Could you check a few things on this model? Use its own coordinates, in mm. A direction names the side the tool comes from. Coordinates: 2 decimals unless noted, no trailing zeros. Order: outer loops, then holes, each group sorted by start corner. A loop starts at its lowest first (then second) coordinate and runs counter-clockwise, first axis right, second up. Notation, with made-up numbers: (75, 29) - (134, 29) arc R16 cw to (134, 44) - close; hole circle Ø3 at (75.25, 69). An arc over 180 degrees is marked (long way). Answer as a JSON object with one key per item and string values. Group by question number.
(1) We'd pull the mould along X, two halves only. Please class faces 1 (the flat face through (-0.775, 16, 1)), 2 (the flat face through (-16, -0.775, 1)), 3 (the cylindrical face through (25.275, 19.38, 0.986)): pulls with the +X half, pulls with the -X half, needs draft (parallel to the pull), parting line crosses it, or undercut.
(2) Imagine slicing it at A-A, the plane x = -7.5. Write out the boundary of the cut face in (y, z) (3 decimals), and give its area (3 significant figures).
(3) Imagine slicing it at B-B, the plane y = 25.5. Write out the boundary of the cut face in (x, z) (3 decimals).
(4) Please list where these lines run through material, in increasing order: probe 1 along Z at (x, y) = (22.5, 26); probe 2 along Z at (x, y) = (-0.5, -31.5); probe 3 along Y at (x, z) = (-28, 1.35) (3 decimals).
(5) Imagine slicing it at C-C, the plane z = 3.5. Write out the boundary of the cut face in (x, y), and give its area (3 significant figures).
(6) Which directions (+Z, -Z, +X, -X, +Y, -Y) give clear straight access to the entire face, cutting with the end or side of a thin tool? Please do faces 4 (the flat face through (-16, 0.775, 1)), 5 (the flat face through (10, 31, 2)), 6 (the flat face through (0.775, 0, 1)).
(7) Will these pins go through, and if not, where does the flat tip stop? P1, Ø1.2, axis at x = -11, z = 0.5, coming from the -Y side; P2, Ø2, axis at x = 27, z = 2, coming from the -Y side; P3, Ø1.2, axis at y = 18, z = 0.5, coming from the +X side.
from build123d import *

# Parameters (mm, degrees)
SKETCH1_R               = 34.5
BOSS_EXTRUDE1_DEPTH     = 4.5
SKETCH2_W               = 2.65
SKETCH2_H               = 2
CUT_EXTRUDE1_DEPTH      = 49.997448913
CUT_EXTRUDE1_DEPTH_BACK = 49.997448913
SKETCH4_W               = 1.55
SKETCH4_H               = 1.5
SKETCH6_W               = 1.5
SKETCH6_H               = 1.55
CUT_EXTRUDE2_DEPTH      = 49.997448913


with BuildPart() as part:
    # Sketch1 → Boss-Extrude1 (new body)
    with BuildSketch(Plane.XY):
        Circle(SKETCH1_R)
    extrude(amount=BOSS_EXTRUDE1_DEPTH)

    # Sketch2 → Cut-Revolve1 (revolve, cut)
    with BuildSketch(Plane(origin=(0, 0, 0), x_dir=(1, 0, 0), z_dir=(0, 1, 0)), mode=Mode.PRIVATE) as cut_revolve1_sk:
        with Locations((33.175, -1)):
            Rectangle(SKETCH2_W, SKETCH2_H)
    revolve(cut_revolve1_sk.sketch.rotate(Axis((0, 0, 0), (0, 0, 1)), 180), axis=Axis((0, 0, 0), (0, 0, 1)), mode=Mode.SUBTRACT)

    # Sketch4 → Cut-Extrude1 (cut, two sides: drawn at the far end of the back side and taken through both)
    with BuildSketch(Plane(origin=(0, 0, 0), x_dir=(1, 0, 0), z_dir=(0, 1, 0)).offset(-CUT_EXTRUDE1_DEPTH_BACK)):
        with Locations((0, -0.75)):
            Rectangle(SKETCH4_W, SKETCH4_H)
    extrude(amount=CUT_EXTRUDE1_DEPTH + CUT_EXTRUDE1_DEPTH_BACK, mode=Mode.SUBTRACT)

    # Sketch6 → Cut-Extrude2 (cut, through all)
    with BuildSketch(Plane(origin=(0, 0, 0), x_dir=(0, 0, -1), z_dir=(1, 0, 0))):
        with Locations((-0.75, 0)):
            Rectangle(SKETCH6_W, SKETCH6_H)
    extrude(amount=-CUT_EXTRUDE2_DEPTH, mode=Mode.SUBTRACT)


solid = part.part
Result set:
{
 "1": {"face 1": "undercut", "face 2": "needs draft", "face 3": "parting line crosses it"},
 "2": {"outline": "(-33.675, 2) - (-30.954, 2) - (-30.954, 0) - (-0.775, 0) - (-0.775, 1.5) - (0.775, 1.5) - (0.775, 0) - (30.954, 0) - (30.954, 2) - (33.675, 2) - (33.675, 4.5) - (-33.675, 4.5) - close", "area": "290 mm^2"},
 "3": {"outline": "(-23.238, 2) - (-19.083, 2) - (-19.083, 0) - (-0.775, 0) - (-0.775, 1.5) - (0.775, 1.5) - (0.775, 0) - (19.083, 0) - (19.083, 2) - (23.238, 2) - (23.238, 4.5) - (-23.238, 4.5) - close"},
 "4": {"probe 1": "z = 2 to 4.5", "probe 2": "z = 1.5 to 4.5", "probe 3": "y = -15.18 to -0.775, 0.775 to 15.18"},
 "5": {"outline": "circle Ø69 at (0, 0)", "area": "3,740 mm^2"},
 "6": {"face 4": "-Z, -X", "face 5": "-Z", "face 6": "-Z, +Y, -Y"},
 "7": {"P1": "stops at y = -30.1", "P2": "stops at y = -22.68", "P3": "stops at x = 26.68"}
}
